Can you work these out from the model? Positions are in its coordinate system, mm. Face numbers are marked on the shaded views. A direction names the side the tool comes from. Give positions to 0.01 mm unless a question says otherwise; leave off trailing zeros. Order: outer loops, then holes, each group sorted by start corner. A loop starts at its lowest first (then second) coordinate and runs counter-clockwise, first axis right, second up. Notation, with made-up numbers: M 15,60 L 21,60 A32 cw 21,90 Z; hole C 22.25,-13 d7. An arc over 180 degrees is marked long. Answer as a JSON object with one key per item and string values.
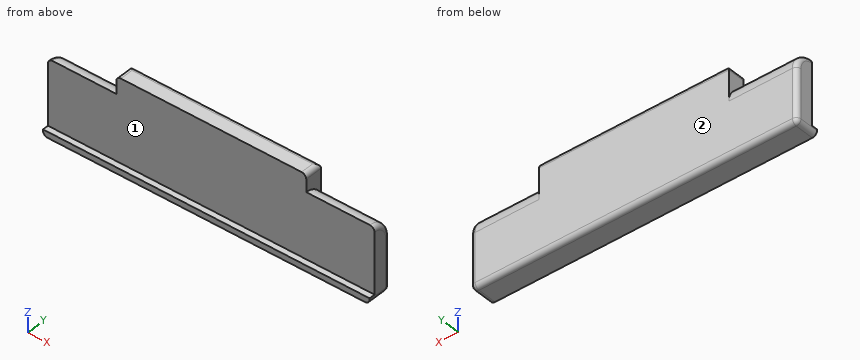
```python
from build123d import *

# Parameters (mm, degrees)
EXTRUDE003_DEPTH = 69.85
BOX024_W         = 40.64
BOX024_H         = 3.81
BOX024_DEPTH     = 7.62
BOX025_W         = 69.85
BOX025_H         = 1.27
BOX025_DEPTH     = 1.27
BOX023_W         = 69.85
BOX023_H         = 3.81
BOX023_DEPTH     = 11.43
FILLET002_R      = 1


with BuildPart() as extrude003:
    # Sketch001 (on Face2 of Box023) → Extrude003 (new body)
    with BuildSketch(Plane.YZ.offset(69.85)):
        with BuildLine():
            ThreePointArc((3.81, 11.43), (2.694077, 14.124077), (0, 15.24))
            Line((0, 15.24), (0, 11.43))
            Line((0, 11.43), (3.81, 11.43))
        make_face()
    extrude(amount=-EXTRUDE003_DEPTH)


with BuildPart() as cube024:
    # Box024 → Box024 (new body)
    with BuildSketch(Plane(origin=(14.605, 0, 11.303), x_dir=(1, 0, 0), z_dir=(0, 0, 1))):
        with Locations((20.32, 1.905)):
            Rectangle(BOX024_W, BOX024_H)
    extrude(amount=BOX024_DEPTH)


with BuildPart() as cube025:
    # Box025 → Box025 (new body)
    with BuildSketch(Plane(origin=(0, -1.27, 0), x_dir=(1, 0, 0), z_dir=(0, 0, 1))):
        with Locations((34.925, 0.635)):
            Rectangle(BOX025_W, BOX025_H)
    extrude(amount=BOX025_DEPTH)


with BuildPart() as fillet002:
    # Box023 → Box023 (new body)
    with BuildSketch(Plane.XY):
        with Locations((34.925, 1.905)):
            Rectangle(BOX023_W, BOX023_H)
    extrude(amount=BOX023_DEPTH)

    # Fusion019: union Extrude003, Cube024, Cube025
    add(extrude003.part)
    add(cube024.part)
    add(cube025.part)

    # Fillet002
    fillet002_edges = [fillet002.edges().sort_by_distance(p)[0] for p in [
        (0, 3.81, 5.715),
        (0, 1.905, 0),
        (0, -0.635, 0),
        (0, 2.694077, 14.124077),
        (69.85, 3.81, 5.715),
        (34.925, 3.81, 0),
        (69.85, 1.905, 0),
        (69.85, -0.635, 0),
        (69.85, 2.694077, 14.124077),
        (14.605, 1.905, 18.923),
        (55.245, 1.905, 18.923),
        (34.925, 3.81, 18.923),
    ]]
    fillet(fillet002_edges, radius=FILLET002_R)


with BuildPart() as fillet002_1:
    # Fillet002 placement: moved
    add(fillet002.part.moved(Location((63.5, -27.94, 0))))


solid = fillet002_1.part
```
1) I want a section at C-C on x = 127.5. Write out the boundary of the cut face in (y, z).
Results found:
{"outline": "M -29.21,0 L -25.13,0 A1 ccw -24.13,1 L -24.13,11.43 A3.81 ccw -27.94,15.24 L -27.94,1.27 L -29.21,1.27 Z"}
2) I want a section at B-B on z = 9.75. Write out the boundary of the cut face in (x, y).
Results found:
{"outline": "M 63.5,-27.94 L 133.35,-27.94 L 133.35,-25.13 A1 ccw 132.35,-24.13 L 64.5,-24.13 A1 ccw 63.5,-25.13 Z"}
3) I want a section at A-A on x = 98. Write out the boundary of the cut face in (y, z), and give its area (3 significant figures).
Results found:
{"outline": "M -29.21,0 L -25.13,0 A1 ccw -24.13,1 L -24.13,17.92 A1 ccw -25.13,18.92 L -27.94,18.92 L -27.94,1.27 L -29.21,1.27 Z", "area": "73.3 mm²"}
4) I'm going to push flat-ended pins straight in: pin 1 Ø3 at (x, z) = (125, 12.5) entering from -Y; pin 2 Ø0.6 at (x, y) = (84.5, -28.5) entering from +Z; pin 3 Ø1 at (y, z) = (-26, 14.5) entering from +X. Where does each tip first touch, or does it pass through?
Results found:
{"pin 1": "stops at y = -27.94", "pin 2": "stops at z = 1.27", "pin 3": "stops at x = 133.3"}
5) I want a section at D-D on z = 16.75. Write out the boundary of the cut face in (x, y) (3 decimals).
Results found:
{"outline": "M 78.105,-27.94 L 118.745,-27.94 L 118.745,-24.13 L 78.105,-24.13 Z"}
6) For the marked faces 1 and 2, which set-ups out of +Z, -Z, +X, -X, +Y, -Y let a thin tool reach every point of the face, with its end or its side?
Results found:
{"face 1": "+Z, +X, -X, -Y", "face 2": "+Z, -Z, +X, -X, +Y"}
7) I need wall thicknesses on L1, parallel to Y at x = 102, z = 13; L2, parallel to Z at x = 75, y = -28.9; L3, parallel to X at y = -25, z = 1.5. Which ranges of each line are inside material? Lowest first, please.
Results found:
{"L1": "y = -27.94 to -24.13", "L2": "z = 0 to 1.27", "L3": "x = 63.51 to 133.34"}
